Design review of the part built by this model. Coordinates are the model's own, in mm. A direction names the side the tool comes from. Round coordinates to 2 decimals unless told otherwise and drop trailing zeros. Write each loop counter-clockwise with the first axis right and the second up, starting at its lowest first coordinate (ties: lowest second). Pieces come first, ordered by that corner, then holes. Notation, with made-up numbers: M 75,47 L 122,47 A11 cw 122,60 Z; hole C 49,60.5 d11. An arc over 180 degrees is marked long. Use CSV: the item, a comma, the result in double quotes.
from build123d import *

# Parameters (mm, degrees)
SKETCH1_W           = 57
SKETCH1_H           = 44
SKETCH1_R           = 1.75
SKETCH1_R_2         = 3
BOSS_EXTRUDE1_DEPTH = 8.1
SKETCH2_R           = 19.65
CUT_EXTRUDE1_DEPTH  = 4
SKETCH3_R           = 3
CUT_EXTRUDE2_DEPTH  = 1.5
FILLET2_R           = 3.5
SKETCH10_W          = 1
SKETCH10_H          = 1.6


with BuildPart() as part:
    # Sketch1 → Boss-Extrude1 (new body)
    with BuildSketch(Plane.XY):
        Rectangle(SKETCH1_W, SKETCH1_H)
        Circle(SKETCH1_R, mode=Mode.SUBTRACT)
        with Locations((-9.5, 0)):
            Circle(SKETCH1_R_2, mode=Mode.SUBTRACT)
        with Locations((9.5, 0)):
            Circle(SKETCH1_R_2, mode=Mode.SUBTRACT)
    extrude(amount=BOSS_EXTRUDE1_DEPTH)

    # Sketch2 → Cut-Extrude1 (cut)
    with BuildSketch(Plane.XY.offset(8.1)):
        Circle(SKETCH2_R)
    extrude(amount=-CUT_EXTRUDE1_DEPTH, mode=Mode.SUBTRACT)

    # Sketch3 → Cut-Extrude2 (cut)
    with BuildSketch(Plane.XY.offset(4.1)):
        Circle(SKETCH3_R)
    extrude(amount=-CUT_EXTRUDE2_DEPTH, mode=Mode.SUBTRACT)

    # Sketch4 → Cut-Revolve1 (revolve, cut)
    with BuildSketch(Plane(origin=(0, 0, 0), x_dir=(1, 0, 0), z_dir=(0, 1, 0))):
        Polygon((0, -2.6), (0, -1.1), (3, -2.6), align=None)
    revolve(axis=Axis((0, 0, 2.6), (0, 0, -1)), mode=Mode.SUBTRACT)

    # Fillet2
    fillet2_edges = [part.edges().sort_by_distance(p)[0] for p in [
        (28.5, -22, 4.05),
        (-28.5, -22, 4.05),
        (-28.5, 22, 4.05),
        (28.5, 22, 4.05),
    ]]
    fillet(fillet2_edges, radius=FILLET2_R)

    # Cut-Sweep1: sweep along a path in Sketch8
    with BuildLine(Plane.XY.offset(8.1)) as cut_sweep1_path:
        Line((25, 22), (-25, 22))
        ThreePointArc((-25, 22), (-27.474873734, 20.974873734), (-28.5, 18.5))
        Line((-28.5, 18.5), (-28.5, -18.5))
        ThreePointArc((-28.5, -18.5), (-27.474873734, -20.974873734), (-25, -22))
        Line((-25, -22), (25, -22))
        ThreePointArc((25, -22), (27.474873734, -20.974873734), (28.5, -18.5))
        Line((28.5, -18.5), (28.5, 18.5))
        ThreePointArc((28.5, 18.5), (27.474873734, 20.974873734), (25, 22))
    # Sketch10 → Cut-Sweep1 (sweep, cut)
    with BuildSketch(Plane(origin=(0, 0, 0), x_dir=(1, 0, 0), z_dir=(0, 1, 0))):
        with Locations((-28, -7.3)):
            Rectangle(SKETCH10_W, SKETCH10_H)
    sweep(path=cut_sweep1_path.line, mode=Mode.SUBTRACT)


solid = part.part
1) The part is to be moulded in two halves that separate along X. For faces 4 (the face through (-27.5, 0, 7)), 5 (the face through (28.5, 0, 3)), 6 (the face through (0, 22, 3)), 7 (the face through (-2.558, 19.483, 6.128)), say which applies: released by +X, released by -X, zero draft, split by the parting line, or undercut.
Answers:
face 4,"released by -X"
face 5,"released by +X"
face 6,"zero draft"
face 7,"undercut"
2) For pin 1 Ø0.8 at (x, z) = (9, 7.5) entering from -Y; pin 2 Ø1.8 at (x, z) = (2.5, 7.5) entering from +Y; pin 3 Ø1.8 at (y, z) = (-6, 7.5) entering from +X, all flat-tipped, find the tip position at first contact; note any pin that passes through.
Answers:
pin 1,"y = -21"
pin 2,"y = 21"
pin 3,"x = 27.5"
3) Add section C-C on z = 1.25. Write out the cut boundary in (x, y).
Answers:
outline,"M -28.5,-18.5 A3.5 ccw -25,-22 L 25,-22 A3.5 ccw 28.5,-18.5 L 28.5,18.5 A3.5 ccw 25,22 L -25,22 A3.5 ccw -28.5,18.5 Z; hole C -9.5,0 d6; hole C 0,0 d3.5; hole C 9.5,0 d6"
4) Add section D-D on x = -11.5. Write out the cut boundary in (y, z).
Answers:
outline,"M -22,0 L -2.24,0 L -2.24,4.1 L -15.93,4.1 L -15.93,8.1 L -21,8.1 L -21,6.5 L -22,6.5 Z; M 2.24,0 L 22,0 L 22,6.5 L 21,6.5 L 21,8.1 L 15.93,8.1 L 15.93,4.1 L 2.24,4.1 Z"
5) Wall thickness on line 1 along X through (y, z) = (0, 1.8); line 2 along Y through (x, z) = (-9.5, 2.6); line 3 along Y through (x, z) = (0, 6.3): over which ranges is each line inside the solid? List them lowest first. Write a range as [from, to].
Answers:
line 1,"[-28.5, -12.5], [-6.5, -1.75], [1.75, 6.5], [12.5, 28.5]"
line 2,"[-22, -3], [3, 22]"
line 3,"[-22, -19.65], [19.65, 22]"
6) Add section B-B on x = 0. Write out the cut boundary in (y, z) (3 decimals).
Answers:
outline,"M -22,0 L -1.75,0 L -1.75,1.975 L -3,2.6 L -3,4.1 L -19.65,4.1 L -19.65,8.1 L -21,8.1 L -21,6.5 L -22,6.5 Z; M 1.75,0 L 22,0 L 22,6.5 L 21,6.5 L 21,8.1 L 19.65,8.1 L 19.65,4.1 L 3,4.1 L 3,2.6 L 1.75,1.975 Z"
7) Add section A-A on y = 0. Write out the cut boundary in (x, z) (3 decimals), then the cut area to 3 significant figures.
Answers:
outline,"M -28.5,0 L -12.5,0 L -12.5,4.1 L -19.65,4.1 L -19.65,8.1 L -27.5,8.1 L -27.5,6.5 L -28.5,6.5 Z; M -6.5,0 L -1.75,0 L -1.75,1.975 L -3,2.6 L -3,4.1 L -6.5,4.1 Z; M 1.75,0 L 6.5,0 L 6.5,4.1 L 3,4.1 L 3,2.6 L 1.75,1.975 Z; M 12.5,0 L 28.5,0 L 28.5,6.5 L 27.5,6.5 L 27.5,8.1 L 19.65,8.1 L 19.65,4.1 L 12.5,4.1 Z"
area,"233 mm²"
8) Machinability: for faces 1 (the face through (-3, 0, 3)), 2 (the face through (-27, 20, 7)), 3 (the face through (0, 21, 7)), which of the approach directions +Z, -Z, +X, -X, +Y, -Y give a long, thin tool a straight path to every point of the face, cutting with its end or side? Answer none if there is none.
Answers:
face 1,"+Z"
face 2,"+Z, -X, +Y"
face 3,"+Z, +X, -X, +Y"
